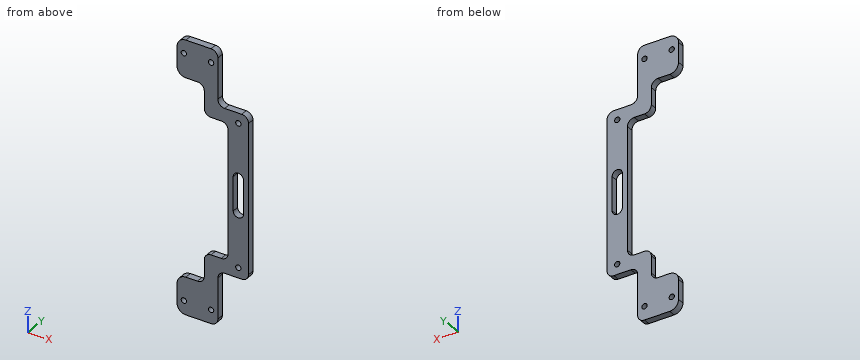
```python
from build123d import *

# Parameters (mm, degrees)
SKETCH1_R           = 2.4892
BOSS_EXTRUDE1_DEPTH = 3.175
FILLET1_R           = 6.35
LPATTERN1_START     = -3.175
LPATTERN1_OUTLINE_R = 2.4892
LPATTERN1_DEPTH     = 6.35
SKETCH2_R           = 2.4892
SKETCH2_W           = 193.675
SKETCH2_H           = 254
CUT_EXTRUDE1_DEPTH  = 344.912740568
FILLET2_R           = 8.255


# Read off the part's stored shape, not the designer's step: LPattern1
with BuildPart() as part:
    # Sketch1 → Boss-Extrude1 (new, symmetric)
    with BuildSketch(Plane(origin=(0, 0, 0), x_dir=(1, 0, 0), z_dir=(0, 1, 0))):
        Polygon((0, 50.8), (0, 0), (203.2, 0), (203.2, 50.8), (231.775, 50.8), (231.775, 203.2), (203.2, 203.2), (203.2, 254), (0, 254), (0, 203.2), (-28.575, 203.2), (-28.575, 50.8), align=None)
        with Locations(Location((196.85, 12.7, 0), (0, 0, 270))):
            Circle(SKETCH1_R, mode=Mode.SUBTRACT)
        Polygon((12.7, 190.5), (12.7, 219.075), (190.5, 219.075), (190.5, 190.5), (212.725, 190.5), (212.725, 63.5), (190.5, 63.5), (190.5, 34.925), (12.7, 34.925), (12.7, 63.5), (-9.525, 63.5), (-9.525, 190.5), align=None, mode=Mode.SUBTRACT)
        with BuildLine():
            Line((227.0125, 142.875), (227.0125, 111.125))
            ThreePointArc((227.0125, 111.125), (222.25, 106.3625), (217.4875, 111.125))
            Line((217.4875, 111.125), (217.4875, 142.875))
            ThreePointArc((217.4875, 142.875), (222.25, 147.6375), (227.0125, 142.875))
        make_face(mode=Mode.SUBTRACT)
        with BuildLine():
            ThreePointArc((-14.2875, 111.125), (-19.05, 106.3625), (-23.8125, 111.125))
            Line((-23.8125, 111.125), (-23.8125, 142.875))
            ThreePointArc((-23.8125, 142.875), (-19.05, 147.6375), (-14.2875, 142.875))
            Line((-14.2875, 142.875), (-14.2875, 111.125))
        make_face(mode=Mode.SUBTRACT)
        with Locations(Location((196.85, 241.3, 0), (0, 0, 270))):
            Circle(SKETCH1_R, mode=Mode.SUBTRACT)
    extrude(amount=BOSS_EXTRUDE1_DEPTH, both=True)

    # Fillet1
    fillet1_edges = [part.edges().sort_by_distance(p)[0] for p in [
        (0, 0, 0),
        (0, 0, -50.8),
        (-28.575, 0, -50.8),
        (-28.575, 0, -203.2),
        (0, 0, -203.2),
        (0, 0, -254),
        (203.2, 0, -254),
        (203.2, 0, -203.2),
        (231.775, 0, -203.2),
        (231.775, 0, -50.8),
        (203.2, 0, -50.8),
        (203.2, 0, 0),
        (212.725, 0, -190.5),
        (190.5, 0, -190.5),
        (190.5, 0, -219.075),
        (12.7, 0, -219.075),
        (12.7, 0, -190.5),
        (-9.525, 0, -190.5),
        (-9.525, 0, -63.5),
        (12.7, 0, -63.5),
        (12.7, 0, -34.925),
        (190.5, 0, -34.925),
        (190.5, 0, -63.5),
        (212.725, 0, -63.5),
    ]]
    fillet(fillet1_edges, radius=FILLET1_R)

    # LPattern1 outline → LPattern1 (cut)
    with BuildSketch(Plane(origin=(0, 0, 0), x_dir=(1, 0, 0), z_dir=(0, 1, 0)).offset(LPATTERN1_START)):
        with Locations((19.05, 12.7)):
            Circle(LPATTERN1_OUTLINE_R)
        with Locations((19.05, 241.3)):
            Circle(LPATTERN1_OUTLINE_R)
        with Locations((44.45, 12.7)):
            Circle(LPATTERN1_OUTLINE_R)
        with Locations((44.45, 241.3)):
            Circle(LPATTERN1_OUTLINE_R)
        with Locations((69.85, 12.7)):
            Circle(LPATTERN1_OUTLINE_R)
        with Locations((69.85, 241.3)):
            Circle(LPATTERN1_OUTLINE_R)
        with Locations((95.25, 12.7)):
            Circle(LPATTERN1_OUTLINE_R)
        with Locations((95.25, 241.3)):
            Circle(LPATTERN1_OUTLINE_R)
        with Locations((120.65, 12.7)):
            Circle(LPATTERN1_OUTLINE_R)
        with Locations((120.65, 241.3)):
            Circle(LPATTERN1_OUTLINE_R)
        with Locations((146.05, 12.7)):
            Circle(LPATTERN1_OUTLINE_R)
        with Locations((146.05, 241.3)):
            Circle(LPATTERN1_OUTLINE_R)
        with Locations((171.45, 12.7)):
            Circle(LPATTERN1_OUTLINE_R)
        with Locations((171.45, 241.3)):
            Circle(LPATTERN1_OUTLINE_R)
    extrude(amount=LPATTERN1_DEPTH, mode=Mode.SUBTRACT)

    # Sketch2 → Cut-Extrude1 (cut, through all)
    with BuildSketch(Plane(origin=(0, 3.175, 0), x_dir=(1, 0, 0), z_dir=(0, 1, 0))):
        with Locations(Location((222.25, 193.675, 0), (0, 0, 270))):
            Circle(SKETCH2_R)
        with Locations(Location((222.25, 60.325, 0), (0, 0, 270))):
            Circle(SKETCH2_R)
        with Locations((68.2625, 127)):
            Rectangle(SKETCH2_W, SKETCH2_H)
    extrude(amount=-CUT_EXTRUDE1_DEPTH, mode=Mode.SUBTRACT)

    # Fillet2
    fillet2_edges = [part.edges().sort_by_distance(p)[0] for p in [
        (165.1, 0, -34.925),
        (165.1, 0, -219.075),
        (165.1, 0, -254),
        (165.1, 0, 0),
    ]]
    fillet(fillet2_edges, radius=FILLET2_R)


solid = part.part
```
Read the model definition and answer for the solid it produces. Units are mm, in the model's axes. Coordinates: 2 decimals unless noted, no trailing zeros. Loops run counter-clockwise (first coordinate to the right, second up) from the corner with the lowest first, then second, coordinate; pieces in that order, holes last. Notation, with made-up numbers: (50, 48) -> (57, 48) arc R27 cw to (57, 82) -> close; hole circle Ø1 at (72.25, -13.5). An arc over 180 degrees is marked (long way). Return JSON: item names as keys, results as strings.
Item 1: Find section B-B (x = 180.5). Determine the outline of the cut face in (y, z) (3 decimals).
Answers:
{"outline": "(-3.175, -254) -> (3.175, -254) -> (3.175, -219.075) -> (-3.175, -219.075) -> close; (-3.175, -34.925) -> (3.175, -34.925) -> (3.175, 0) -> (-3.175, 0) -> close"}
Item 2: Find section D-D (y = 0.5). Count the separate pieces of the cut face and the enclosed holes in it, plus the area to 3 significant figures.
Answers:
{"separate pieces": "1", "enclosed holes": "7", "area": "5,980 mm2"}
Item 3: Flat-ended cylindrical pins translate along their axes: P1, Ø1.5, axis at x = 206, y = 1, coming from the -Z side; P2, Ø3, axis at y = 0, z = -221.5, coming from the +X side; P3, Ø3, axis at x = 202.5, y = -1, coming from the -Z side. Find the tip coordinate at first contact, or state that the pin passes through.
Answers:
{"P1": "stops at z = -204.88", "P2": "stops at x = 203.2", "P3": "stops at z = -252.46"}
Item 4: Find section C-C (x = 222.25). Determine the outline of the cut face in (y, z) (1 decimal).
Answers:
{"outline": "(-3.2, -203.2) -> (3.2, -203.2) -> (3.2, -196.2) -> (-3.2, -196.2) -> close; (-3.2, -191.2) -> (3.2, -191.2) -> (3.2, -147.6) -> (-3.2, -147.6) -> close; (-3.2, -106.4) -> (3.2, -106.4) -> (3.2, -62.8) -> (-3.2, -62.8) -> close; (-3.2, -57.8) -> (3.2, -57.8) -> (3.2, -50.8) -> (-3.2, -50.8) -> close"}
Item 5: Find section A-A (z = -241.3). Determine the outline of the cut face in (x, y) (3 decimals), plus the area to 3 significant figures.
Answers:
{"outline": "(165.1, -3.175) -> (168.961, -3.175) -> (168.961, 3.175) -> (165.1, 3.175) -> close; (173.939, -3.175) -> (194.361, -3.175) -> (194.361, 3.175) -> (173.939, 3.175) -> close; (199.339, -3.175) -> (203.2, -3.175) -> (203.2, 3.175) -> (199.339, 3.175) -> close", "area": "179 mm2"}
Item 6: Find the intervals of material crossed by probe 1 along X at (y, z) = (-1.5, -241.3); probe 2 along Z at (x, y) = (222.25, 0.5); probe 3 along Z at (x, y) = (196.85, -0.75), in increasing order.
Answers:
{"probe 1": "x = 165.1 to 168.96, 173.94 to 194.36, 199.34 to 203.2", "probe 2": "z = -203.2 to -196.16, -191.19 to -147.64, -106.36 to -62.81, -57.84 to -50.8", "probe 3": "z = -254 to -243.79, -238.81 to -190.5, -63.5 to -15.19, -10.21 to 0"}
